Geometry check sheet. Reference: the model listing, model coordinates, mm. Face numbers are marked on the shaded views. Coordinates: 2 decimals unless noted, no trailing zeros. Loops run counter-clockwise (first coordinate to the right, second up) from the corner with the lowest first, then second, coordinate; pieces in that order, holes last.
from build123d import *

# Parameters (mm, degrees)
F1_DEPTH = 25.4
F2_SIZE  = 12.7
F3_R     = 29.887927


with BuildPart() as f1:
    # F0 (on Front) → F1 (new body)
    with BuildSketch(Plane.XZ):
        Polygon((53.427204, 36.90131), (-46.108402, 36.90131), (0, -45.14505), align=None)
    extrude(amount=F1_DEPTH)

    # F2
    f2_edges = [f1.edges().sort_by_distance(p)[0] for p in [
        (-46.108402, -12.7, 36.90131),
    ]]
    chamfer(f2_edges, length=F2_SIZE)

    # F3
    f3_edges = [f1.edges().sort_by_distance(p)[0] for p in [
        (0, -12.7, -45.14505),
    ]]
    fillet(f3_edges, radius=F3_R)


solid = f1.part
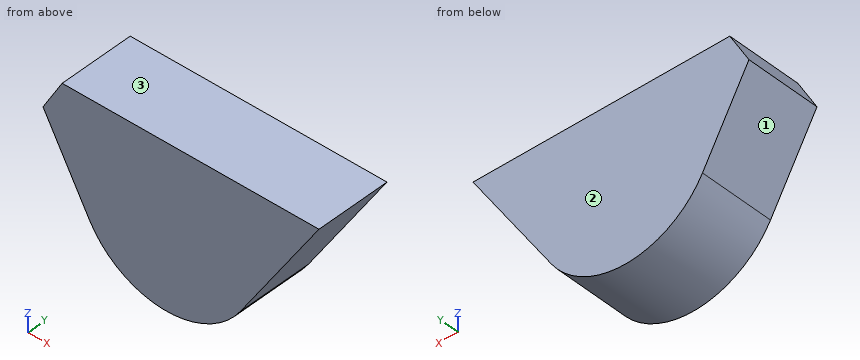
1) Section check A-A on y = -2.75. Record the cut outline in (x, z), and give its area (3 significant figures).
Data:
outline: (-39.89, 25.83) - (-24.17, -2.13) arc R29.89 ccw to (26.93, -3.79) - (53.43, 36.9) - (-33.41, 36.9) - close
area: 3,450 mm2
2) Material ranges on probe 1 along Z at (x, y) = (1.5, -15.5); probe 2 along X at (y, z) = (-11.75, -3); probe 3 along Z at (x, y) = (26.5, -13.25), recorded low to high.
Data:
probe 1: z = -17.37 to 36.9
probe 2: x = -23.67 to 27.44
probe 3: z = -4.43 to 36.9
3) Depth check by flat-ended pin: pin 1 (3 mm diameter, centred on x = -1, y = -4.5, fed in from -Z); pin 2 (1.5 mm diameter, centred on y = -13, z = 12, fed in from +X); pin 3 (5 mm diameter, centred on x = -4.5, y = -2.5, fed in from -Z). Enter the tip coordinate at first touch or a pass-through.
Data:
pin 1: stops at z = -17.34
pin 2: stops at x = 37.7
pin 3: stops at z = -17.12
4) Section check B-B on x = -21. Record the cut outline in (y, z).
Data:
outline: (-25.4, -6.71) - (0, -6.71) - (0, 36.9) - (-25.4, 36.9) - close
5) Mould release check, pull along Z, two halves, no side actions. Record for the marked faces 1, 2 and 3: +Z half, -Z half, draft (parallel to the pull), parting line (faces both ways), or undercut.
Data:
face 1: -Z half
face 2: draft
face 3: +Z half
6) Section check C-C on z = 20.5. Record the cut outline in (x, y), and give its area (3 significant figures).
Data:
outline: (-36.89, -25.4) - (42.75, -25.4) - (42.75, 0) - (-36.89, 0) - close
area: 2,020 mm2
